Check sheet for the modelled part. Datum: model origin and axes. Units: mm. Coordinates: 2 decimals unless noted, no trailing zeros. Write each loop counter-clockwise with the first axis right and the second up, starting at its lowest first coordinate (ties: lowest second). Pieces come first, ordered by that corner, then holes. Notation, with made-up numbers: (32.25, 3) - (83.25, 3) arc R32 ccw to (83.25, 36) - close; hole circle Ø6 at (59, 17.5). An arc over 180 degrees is marked (long way). Answer as CSV lines item,"result". Start each with the question number.
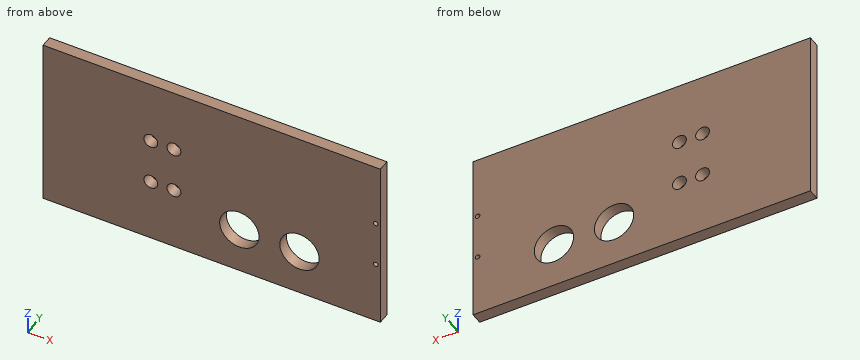
Autodesk Inventor part; units mm, degrees
ref_plane "YZ Plane" through (0, 0, 0) normal (1, 0, 0) x (0, 1, 0)
ref_plane "XZ Plane" through (0, 0, 0) normal (0, 1, 0) x (-1, 0, 0)
ref_plane "XY Plane" through (0, 0, 0) normal (0, 0, 1) x (1, 0, 0)
sketch "Sketch1" plane through (0, 0, 0) normal (0, 0, 1) x (1, 0, 0)
  line L0 (0, 0) -> (145.9214, 0)
  line L1 (145.9214, 0) -> (145.9214, 5)
  line L2 (145.9214, 5) -> (0, 5)
  line L3 (0, 5) -> (0, 0)
  dimension "d0" = 145.9214
  dimension "d1" = 5
extrude "Extrusion1" add sketch "Sketch1" along normal blind 75
sketch "Sketch2" plane through (0, 0, 0) normal (0, -1, 0) x (1, 0, 0)
  circle A0 centre (46.6338, 27.5) radius 3
  line L0 (0, 0) -> (145.9214, 0)
  line L1 (0, 0) -> (0, 75)
  circle A1 centre (46.6338, 47.5) radius 3
  circle A2 centre (56.6338, 47.5) radius 3
  circle A3 centre (56.6338, 27.5) radius 3
  dimension "d4" = 6
  dimension "d5" = 27.5
  dimension "d6" = 46.6338
  dimension "d7" = 6
  dimension "d8" = 20
  dimension "d9" = 6
  dimension "d10" = 6
  dimension "d11" = 10
extrude "Extrusion2" cut sketch "Sketch2" against normal through all
sketch "Sketch3" plane through (0, 0, 0) normal (0, -1, 0) x (1, 0, 0)
  circle A0 centre (46.6338, 27.5) radius 3
  circle A1 centre (143.9214, 27.5) radius 1
  circle A2 centre (143.9214, 47.5) radius 1
  circle A3 centre (46.6338, 47.5) radius 3
  line L0 (145.9214, 0) -> (145.9214, 75)
  point P0 (0, 0)
  dimension "d22" = 2
  dimension "d23" = 2
  dimension "d24" = 2
extrude "Extrusion3" cut sketch "Sketch3" against normal through all contours A1 | A2
thread "Thread7"
thread "Thread8"
sketch "Sketch4" plane through (0, 0, 0) normal (0, -1, 0) x (1, 0, 0)
  circle A0 centre (110.9214, 20) radius 8.5
  line L0 (145.9214, 0) -> (145.9214, 75)
  line L1 (0, 75) -> (145.9214, 75)
  circle A1 centre (84.9214, 20) radius 8.5
  point P0 (0, 0)
  dimension "d35" = 17
  dimension "d36" = 35
  dimension "d38" = 17
  dimension "d39" = 26
  dimension "d42" = 20
extrude "Extrusion4" cut sketch "Sketch4" against normal through all
properties part number "CW001" material "ABS Plastic"
(1) Material ranges on probe 1 along X at (y, z) = (1, 46); probe 2 along X at (y, z) = (3.9, 25); probe 3 along X at (y, z) = (0.85, 19), recorded low to high. Write a range as from..to.
(2) Cross-section at A-A on z = 20. Record the boundary of the cut face in (x, y), plus the area to 3 significant figures.
(3) Cross-section at B-B on y = 0.95. State how many separate pieces and enclosed holes the cut face has, plus the area to 3 significant figures.
Checked values:
1,probe 1,"0..44.04, 49.23..54.04, 59.23..145.92"
1,probe 2,"0..44.98, 48.29..54.98, 58.29..78.05, 91.8..104.05, 117.8..145.92"
1,probe 3,"0..76.48, 93.36..102.48, 119.36..145.92"
2,outline,"(0, 0) - (76.42, 0) - (76.42, 5) - (0, 5) - close; (93.42, 0) - (102.42, 0) - (102.42, 5) - (93.42, 5) - close; (119.42, 0) - (145.92, 0) - (145.92, 5) - (119.42, 5) - close"
2,area,"560 mm^2"
3,separate pieces,"1"
3,enclosed holes,"8"
3,area,"10,400 mm^2"
